The figure shows three views and two pictorial views of one solid part (mm, origin at its lowest corner). Answer the questions. A direction names the side the tool comes from. Give positions to 0.01 mm unless a question says otherwise; leave off trailing zeros. Order: outer loops, then holes, each group sorted by start corner. A loop starts at its lowest first (then second) coordinate and runs counter-clockwise, first axis right, second up. Notation, with made-up numbers: (24, 79) - (59, 79) arc R26 cw to (59, 95) - close; hole circle Ø1 at (59.5, 32.25). An arc over 180 degrees is marked (long way). Use a Markdown table: item, result. Add a question column.
1. A cutting plane is placed at A-A on z = 343.5. Determine the outline of the cut face in (x, y).
2. Flat-ended cylindrical pins translate along their axes: P1, Ø4, axis at x = 91, y = 27, coming from the +Z side; P2, Ø15, axis at y = 22.5, z = 200.5, coming from the -X side; P3, Ø7.5, axis at x = 53, y = 16, coming from the -Z side. Find the tip coordinate at first contact, or state that the pin passes through.
3. A cutting plane is placed at B-B on y = 14.75. Determine the outline of the cut face in (x, z), and give its area (3 significant figures).
4. Consider L1, parallel to X at y = 27.85, z = 85; L2, parallel to Y at x = 6.5, z = 34. Determine where each line is inside the solid, lowest interval first.
5. Which of the six approach directions +Z, -Z, +X, -X, +Y, -Y give full straight-line access (tool end or side, diameter ignored) to the marked faces 1 and 2?
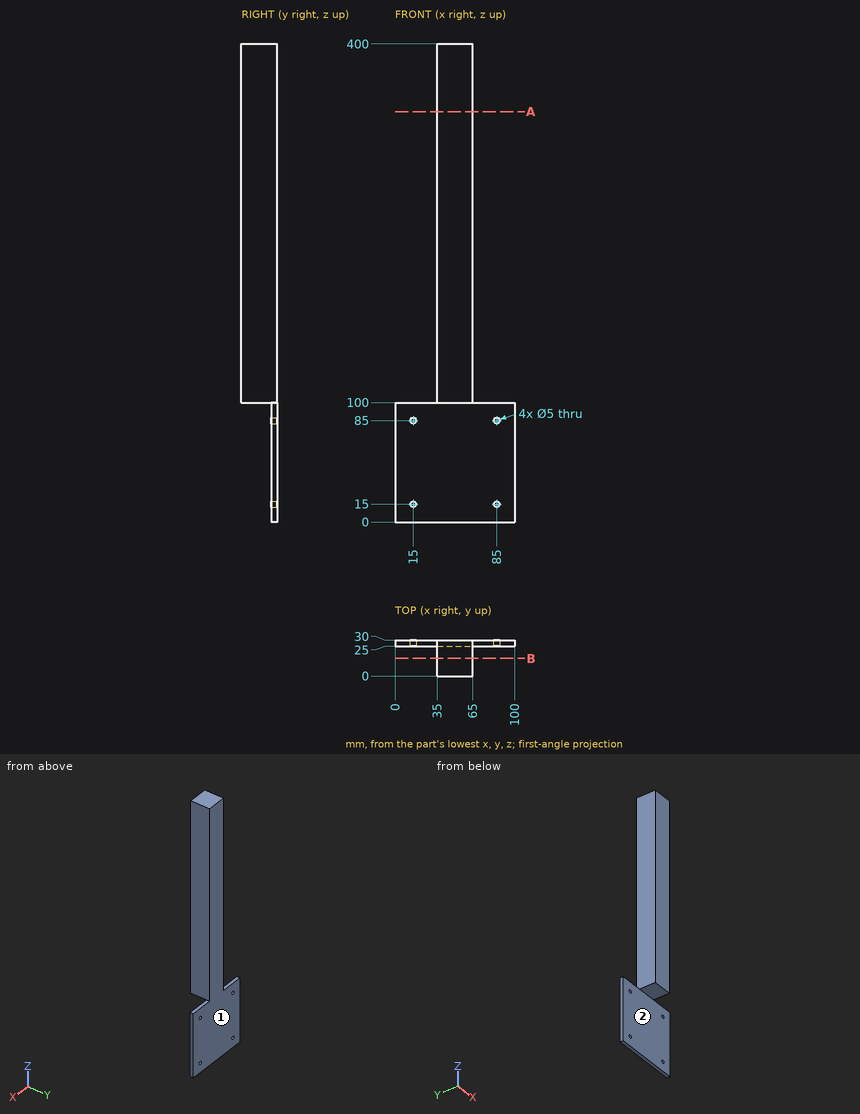
Output values:
| question | item | result |
|---|---|---|
| 1 | outline | (35, 0) - (65, 0) - (65, 30) - (35, 30) - close |
| 2 | P1 | z = 100 |
| 2 | P2 | x = 35 |
| 2 | P3 | z = 100 |
| 3 | outline | (35, 100) - (65, 100) - (65, 400) - (35, 400) - close |
| 3 | area | 9,000 mm² |
| 4 | L1 | 0 to 12.5, 17.5 to 82.5, 87.5 to 100 |
| 4 | L2 | 25 to 30 |
| 5 | face 1 | +Z, -Z, +X, -X, +Y |
| 5 | face 2 | -Z, +X, -X, -Y |
